Can you work these out from the model? Positions are in its coordinate system, mm. A direction names the side the tool comes from. Coordinates: 2 decimals unless noted, no trailing zeros. Order: outer loops, then holes, each group sorted by start corner. A loop starts at its lowest first (then second) coordinate and runs counter-clockwise, first axis right, second up.
Solid Edge part; units mm, degrees
sketch "Sketch1" plane through (0, 0, 0) normal (0, -1, 0) x (1, 0, 0)
  line L0 (7.245, 25) -> (7.245, 22)
  line L1 (7.245, 22) -> (1.245, 22)
  line L2 (1.245, 22) -> (1.245, 25)
  line L3 (1.245, 25) -> (-17.075, 25)
  line L4 (-17.075, 25) -> (-17.075, 27)
  line L5 (-17.075, 27) -> (-14.075, 27)
  line L6 (-14.075, 27) -> (-14.075, 29)
  line L7 (-14.075, 29) -> (-21.215, 29)
  line L8 (-21.215, 29) -> (-21.215, 25)
  line L9 (-21.215, 25) -> (-21.215, 18.75)
  line L10 (-10.6075, 0) -> (-21.215, 18.75)
  line L11 (-10.6075, 0) -> (-6.5872, 0)
  line L12 (14.2453, 20) -> (-6.5872, 0)
  line L13 (14.2453, 20) -> (14.2453, 29.9651)
  line L14 (14.2453, 29.9651) -> (9.2448, 29.9651)
  line L15 (9.2448, 25.0006) -> (9.2448, 29.9651)
  line L16 (9.2448, 25.0006) -> (7.245, 25)
  circle A0 centre (-5.7743, 12.842) radius 5
  circle A1 centre (-14.4595, 19.0255) radius 3
  circle A2 centre (4.1767, 17.035) radius 3
  circle A3 centre (11.7453, 27.685) radius 0.685
extrude "Protrusion1" add sketch "Sketch1" along normal blind 2
properties material "Acrylic, high impact grade"
1. I'm going to push flat-ended pins straight in: pin 1 (0.6 mm diameter, centred on x = 4, y = -1.5, fed in from +Z); pin 2 (0.6 mm diameter, centred on x = 8, y = -1.5, fed in from +Z); pin 3 (0.6 mm diameter, centred on x = -15.5, y = -1, fed in from -Z); pin 4 (9 mm diameter, centred on x = -5.77, z = 12.84, fed in from +Y). Where does each tip first touch, or does it pass through?
Completed:
pin 1: stops at z = 22
pin 2: stops at z = 25
pin 3: stops at z = 8.12
pin 4: passes through
2. Please list where these lines run through material, in increasing order: probe 1 along X at (y, z) = (-0.55, 27.75) (3 decimals); probe 2 along X at (y, z) = (-0.1, 25.5) (3 decimals); probe 3 along X at (y, z) = (-1.45, 18.75) (3 decimals).
Completed:
probe 1: x = -21.215 to -14.075, 9.245 to 11.063, 12.427 to 14.245
probe 2: x = -21.215 to -17.075, 9.245 to 14.245
probe 3: x = -21.215 to -17.447, -11.472 to 1.715, 6.638 to 12.943
3. On a 3-axis mill with a long thin cutter (end or side, diameter ignored), from which of +Z, -Z, +X, -X, +Y, -Y can I reach the whole of each face in a straight line? I mean faces 1 (the flat face through (7.245, -1, 24)), 2 (the flat face through (-16, -1, 27)), 3 (the flat face through (3.975, -0.986, 10.14)). Say none if no direction works.
Completed:
face 1: +Z, +Y, -Y
face 2: +Y, -Y
face 3: -Z, +X, +Y, -Y
4. Imagine slicing it at C-C on x = -16.5. Please give me the cut outline in (y, z), then the cut area to 3 significant figures.
Completed:
outline: (-2, 10.42) - (0, 10.42) - (0, 16.83) - (-2, 16.83) - close; (-2, 21.22) - (0, 21.22) - (0, 25) - (-2, 25) - close; (-2, 27) - (0, 27) - (0, 29) - (-2, 29) - close
area: 24.4 mm2
5. Imagine slicing it at D-D on y = -0.6. Give the number of separate pieces and of enclosed holes in the cut face, then the cut area to 3 significant figures.
Completed:
separate pieces: 1
enclosed holes: 4
area: 472 mm2
6. Imagine slicing it at A-A on z = 24. Please give me the cut outline in (x, y) (3 decimals).
Completed:
outline: (-21.215, -2) - (1.245, -2) - (1.245, 0) - (-21.215, 0) - close; (7.245, -2) - (14.245, -2) - (14.245, 0) - (7.245, 0) - close
7. Thinking about a two-plate mould opening in Z: for faces 4 (the flat face through (-9, -1, 0)), 5 (the flat face through (-17.075, -1, 26)), 6 (the flat face through (-18, -1, 29)), 7 (the cylindrical face through (-6.425, -0.986, 7.885)), which applies, pulls with the +Z half, pulls with the -Z half, needs draft (parallel to the pull), parting line crosses it, or undercut?
Completed:
face 4: pulls with the -Z half
face 5: undercut
face 6: pulls with the +Z half
face 7: undercut
8. Imagine slicing it at B-B on x = -7.5. Please give me the cut outline in (y, z), then the cut area to 3 significant figures.
Completed:
outline: (-2, 0) - (0, 0) - (0, 8.15) - (-2, 8.15) - close; (-2, 17.53) - (0, 17.53) - (0, 25) - (-2, 25) - close
area: 31.2 mm2
